Build history of the part. All positions in model axes, mm. A direction names the side the tool comes from. Round coordinates to 2 decimals unless told otherwise and drop trailing zeros. Write each loop counter-clockwise with the first axis right and the second up, starting at its lowest first coordinate (ties: lowest second). Pieces come first, ordered by that corner, then holes. Notation, with made-up numbers: (68, 41) -> (127, 41) arc R18 cw to (127, 51) -> close; hole circle Ø2 at (28.25, -20.75). An arc over 180 degrees is marked (long way). Answer as CSV lines item,"result".
from build123d import *

# Parameters (mm, degrees)
F1_DEPTH = 40


with BuildPart() as f1:
    # F0 (on Top) → F1 (new body)
    with BuildSketch(Plane.XY):
        with BuildLine():
            Line((-170, 40), (-170, 0))
            Line((-170, 0), (-90, 0))
            Line((-90, 0), (-90, 50.562589))
            ThreePointArc((-90, 50.562589), (-85, 95), (-80, 50.562589))
            Line((-80, 50.562589), (-80, 0))
            Line((-80, 0), (0, 0))
            Line((0, 0), (0, 40))
            ThreePointArc((0, 40), (-24.895924, 100.104076), (-85, 125))
            ThreePointArc((-85, 125), (-145.104076, 100.104076), (-170, 40))
        make_face()
    extrude(amount=F1_DEPTH)


solid = f1.part
1. Drop flat-ended pins along their axis: pin 1 Ø1.5 at (y, z) = (41, 26) entering from -X; pin 2 Ø10 at (y, z) = (109, 11.5) entering from -X. Give the stop position or say it passes through.
Results found:
pin 1,"stops at x = -170"
pin 2,"stops at x = -140.94"
2. Which spindle directions (+Z, -Z, +X, -X, +Y, -Y) get a long thin tool onto all of the face, cutting with end or side? Do faces 4 (the flat face through (-80, 26, 20)), 5 (the flat face through (-67, 49, 0)). Say none if no direction does.
Results found:
face 4,"+Z, -Z, -Y"
face 5,"-Z, +X, -X, +Y, -Y"
3. Probe line 1 along Y through (x, z) = (-85, 19); line 2 along X through (y, z) = (72, 23); line 3 along X through (y, z) = (69, 20). List the from-to ranges inside material, lowest first.
Results found:
line 1,"y = 95 to 125"
line 2,"x = -163.75 to -107.49, -62.51 to -6.25"
line 3,"x = -164.9 to -107.23, -62.77 to -5.1"
4. Cut at B-B, the plane x = -96. Write the cut outline in (y, z), then the cut area to 3 significant figures.
Results found:
outline,"(0, 0) -> (52.87, 0) -> (52.87, 40) -> (0, 40) -> close; (92.13, 0) -> (124.29, 0) -> (124.29, 40) -> (92.13, 40) -> close"
area,"3,400 mm2"
5. Cut at D-D, the plane x = -153.5. Write the cut outline in (y, z), then the cut area to 3 significant figures.
Results found:
outline,"(0, 0) -> (90.33, 0) -> (90.33, 40) -> (0, 40) -> close"
area,"3,610 mm2"
6. Cut at A-A, the plane y = 9. Write the cut outline in (x, z), then the cut area to 3 significant figures.
Results found:
outline,"(-170, 0) -> (-90, 0) -> (-90, 40) -> (-170, 40) -> close; (-80, 0) -> (0, 0) -> (0, 40) -> (-80, 40) -> close"
area,"6,400 mm2"
7. Cut at C-C, the plane z = 7. Write the cut outline in (x, y), then the cut area to 3 significant figures.
Results found:
outline,"(-170, 0) -> (-90, 0) -> (-90, 50.56) arc R22.5 cw (long way) to (-80, 50.56) -> (-80, 0) -> (0, 0) -> (0, 40) arc R85 ccw to (-85, 125) arc R85 ccw to (-170, 40) -> close"
area,"16,100 mm2"
8. Mould opens along X. For faces 1 (the flat face through (-41, 0, 20)), 2 (the cylindrical face through (-85.92, 94.98, 19.72)), 3 (the flat face through (-170, 20, 20)) say: +X half, -X half, draft (parallel to the pull), parting line (faces both ways), or undercut.
Results found:
face 1,"draft"
face 2,"undercut"
face 3,"-X half"
